Work out the finished part from the listing and answer in its coordinate system (mm). A direction names the side the tool comes from. Give positions to 0.01 mm unless a question says otherwise; leave off trailing zeros. Write each loop counter-clockwise with the first axis right and the second up, starting at its lowest first coordinate (ties: lowest second). Pieces come first, ordered by that corner, then holes. Notation, with made-up numbers: (65, 15.25) - (95, 15.25) arc R32 cw to (95, 50.25) - close; hole circle Ø1 at (89.5, -37). An arc over 180 degrees is marked (long way). Write item = value, one per line.
from build123d import *

# Parameters (mm, degrees)
PAD_DEPTH       = 25
SKETCH001_W     = 1
SKETCH001_H     = 8
SKETCH001_W_2   = 5
POCKET_DEPTH    = 14
SKETCH002_W     = 12.5
SKETCH002_H     = 8
POCKET001_DEPTH = 1.5
POCKET002_DEPTH = 0.5
SKETCH004_R     = 2
SKETCH004_W     = 0.8
SKETCH004_H     = 3
POCKET003_DEPTH = 8
SKETCH005_R     = 0.7
PAD001_DEPTH    = 2
SKETCH006_R     = 0.7
PAD002_DEPTH    = 2


with BuildPart() as part:
    # Sketch → Pad (new body, symmetric)
    with BuildSketch(Plane.YZ):
        with BuildLine():
            Line((-6, 13.5), (8, 13.5))
            Line((8, 13.5), (8, 0))
            Line((8, 0), (-8, 0))
            Line((-8, 0), (-8, 11.5))
            ThreePointArc((-6, 13.5), (-7.414214, 12.914214), (-8, 11.5))
        make_face()
    extrude(amount=PAD_DEPTH, both=True)

    # Sketch001 (on Face4 of Pad) → Pocket (cut)
    with BuildSketch(Plane(origin=(0, -8, 0), x_dir=(0, 0, -1), z_dir=(0, -1, 0))):
        with Locations((-0.5, -19)):
            Rectangle(SKETCH001_W, SKETCH001_H)
        with Locations((-0.5, -9.5)):
            Rectangle(SKETCH001_W, SKETCH001_H)
        with Locations((-0.5, 0)):
            Rectangle(SKETCH001_W, SKETCH001_H)
        with Locations((-0.5, 9.5)):
            Rectangle(SKETCH001_W, SKETCH001_H)
        with Locations((-0.5, 19)):
            Rectangle(SKETCH001_W, SKETCH001_H)
        with Locations((-11, -19)):
            Rectangle(SKETCH001_W_2, SKETCH001_H)
        with Locations((-11, -9.5)):
            Rectangle(SKETCH001_W_2, SKETCH001_H)
        with Locations((-11, 0)):
            Rectangle(SKETCH001_W_2, SKETCH001_H)
        with Locations((-11, 9.5)):
            Rectangle(SKETCH001_W_2, SKETCH001_H)
        with Locations((-11, 19)):
            Rectangle(SKETCH001_W_2, SKETCH001_H)
    extrude(amount=-POCKET_DEPTH, mode=Mode.SUBTRACT)

    # Sketch002 (on Face3 of Pocket) → Pocket001 (cut)
    with BuildSketch(Plane.ZX.offset(8)):
        with Locations((6.25, 19)):
            Rectangle(SKETCH002_W, SKETCH002_H)
        with Locations((6.25, 9.5)):
            Rectangle(SKETCH002_W, SKETCH002_H)
        with Locations((6.25, 0)):
            Rectangle(SKETCH002_W, SKETCH002_H)
        with Locations((6.25, -9.5)):
            Rectangle(SKETCH002_W, SKETCH002_H)
        with Locations((6.25, -19)):
            Rectangle(SKETCH002_W, SKETCH002_H)
    extrude(amount=-POCKET001_DEPTH, mode=Mode.SUBTRACT)

    # Sketch003 (on Face67 of Pocket001) → Pocket002 (cut)
    with BuildSketch(Plane.ZX.offset(6.5)):
        Polygon((0, 23), (8.5, 23), (8.5, 21.5), (9.5, 21.5), (9.5, 16.5), (8.5, 16.5), (8.5, 15), (0, 15), align=None)
        Polygon((0, 13.5), (8.5, 13.5), (8.5, 12), (9.5, 12), (9.5, 7), (8.5, 7), (8.5, 5.5), (0, 5.5), align=None)
        Polygon((0, 4), (8.5, 4), (8.5, 2.5), (9.5, 2.5), (9.5, -2.5), (8.5, -2.5), (8.5, -4), (0, -4), align=None)
        Polygon((0, -5.5), (8.5, -5.5), (8.5, -7), (9.5, -7), (9.5, -12), (8.5, -12), (8.5, -13.5), (0, -13.5), align=None)
        Polygon((0, -15), (8.5, -15), (8.5, -16.5), (9.5, -16.5), (9.5, -21.5), (8.5, -21.5), (8.5, -23), (0, -23), align=None)
    extrude(amount=-POCKET002_DEPTH, mode=Mode.SUBTRACT)

    # Sketch004 (on Face64 of Pocket002) → Pocket003 (cut)
    with BuildSketch(Plane(origin=(0, 0, 8.5), x_dir=(0, -1, 0), z_dir=(0, 0, 1))):
        with Locations((1.05, -19)):
            Circle(SKETCH004_R)
        with Locations((1.05, -9.5)):
            Circle(SKETCH004_R)
        with Locations((1.05, 0)):
            Circle(SKETCH004_R)
        with Locations((1.05, 9.5)):
            Circle(SKETCH004_R)
        with Locations((1.05, 19)):
            Circle(SKETCH004_R)
        with Locations((-4, -19)):
            Rectangle(SKETCH004_W, SKETCH004_H)
        with Locations((-4, -9.5)):
            Rectangle(SKETCH004_W, SKETCH004_H)
        with Locations((-4, 0)):
            Rectangle(SKETCH004_W, SKETCH004_H)
        with Locations((-4, 9.5)):
            Rectangle(SKETCH004_W, SKETCH004_H)
        with Locations((-4, 19)):
            Rectangle(SKETCH004_W, SKETCH004_H)
        with Locations((6.1, -19)):
            Rectangle(SKETCH004_W, SKETCH004_H)
        with Locations((6.1, -9.5)):
            Rectangle(SKETCH004_W, SKETCH004_H)
        with Locations((6.1, 0)):
            Rectangle(SKETCH004_W, SKETCH004_H)
        with Locations((6.1, 9.5)):
            Rectangle(SKETCH004_W, SKETCH004_H)
        with Locations((6.1, 19)):
            Rectangle(SKETCH004_W, SKETCH004_H)
    extrude(amount=-POCKET003_DEPTH, mode=Mode.SUBTRACT)

    # Sketch005 (on Face2 of Pocket003) → Pad001 (join)
    with BuildSketch(Plane(origin=(-25, 0, 0), x_dir=(0, 1, 0), z_dir=(-1, 0, 0))):
        with BuildLine():
            Line((-6, -13.5), (-2, -13.5))
            Line((-2, -13.5), (-2, -16.3))
            ThreePointArc((-2.7, -17), (-2.205025, -16.794975), (-2, -16.3))
            Line((-2.7, -17), (-5.3, -17))
            ThreePointArc((-6, -16.3), (-5.794975, -16.794975), (-5.3, -17))
            Line((-6, -16.3), (-6, -13.5))
        make_face()
        with Locations((-4, -15.5)):
            Circle(SKETCH005_R, mode=Mode.SUBTRACT)
        with BuildLine():
            Line((4, -13.5), (8, -13.5))
            Line((8, -13.5), (8, -16.3))
            ThreePointArc((7.3, -17), (7.794975, -16.794975), (8, -16.3))
            Line((7.3, -17), (4.7, -17))
            ThreePointArc((4, -16.3), (4.205025, -16.794975), (4.7, -17))
            Line((4, -16.3), (4, -13.5))
        make_face()
        with Locations((6, -15.5)):
            Circle(SKETCH005_R, mode=Mode.SUBTRACT)
    extrude(amount=-PAD001_DEPTH)

    # Sketch006 (on Face4 of Pocket003) → Pad002 (join)
    with BuildSketch(Plane(origin=(25, 0, 0), x_dir=(0, 1, 0), z_dir=(-1, 0, 0))):
        with BuildLine():
            Line((-6, -13.5), (-2, -13.5))
            Line((-2, -13.5), (-2, -16.3))
            ThreePointArc((-2.7, -17), (-2.205025, -16.794975), (-2, -16.3))
            Line((-2.7, -17), (-5.3, -17))
            ThreePointArc((-6, -16.3), (-5.794975, -16.794975), (-5.3, -17))
            Line((-6, -16.3), (-6, -13.5))
        make_face()
        with Locations((-4, -15.5)):
            Circle(SKETCH006_R, mode=Mode.SUBTRACT)
        with BuildLine():
            Line((4, -13.5), (8, -13.5))
            Line((8, -13.5), (8, -16.3))
            ThreePointArc((7.3, -17), (7.794975, -16.794975), (8, -16.3))
            Line((7.3, -17), (4.7, -17))
            ThreePointArc((4, -16.3), (4.205025, -16.794975), (4.7, -17))
            Line((4, -16.3), (4, -13.5))
        make_face()
        with Locations((6, -15.5)):
            Circle(SKETCH006_R, mode=Mode.SUBTRACT)
    extrude(amount=PAD002_DEPTH)


solid = part.part
1. Given pin 1 (2.5 mm diameter, centred on x = -19.5, y = -4, fed in from +Z); pin 2 (3 mm diameter, centred on x = 8.5, y = 4, fed in from -Z); pin 3 (6 mm diameter, centred on x = 0.5, z = 4.5, fed in from +Y), each flat-ended and moving along its own axis, determine where each tip first touches the part or whether it passes through.
Solution:
pin_1 = 8.5
pin_2 = 1
pin_3 = 6
2. Find section D-D, the plane z = 6.75. Give the number of separate pieces and of enclosed holes in the cut face, then the cut area to 3 significant figures.
Solution:
separate_pieces = 1
enclosed_holes = 15
area = 633 mm^2
3. A tool of negligible diameter and unlimited length cuts with its end or side. For faces 1 (the flat face through (15, 7, 3)), 2 (the flat face through (9, 4.4, 5)), 3 (the flat face through (15, -1, 11)), 4 (the flat face through (7.7, 0.5, 1)), from which of +Z, -Z, +X, -X, +Y, -Y can it reach the whole face along a straight path? Write none if from no direction.
Solution:
face_1 = -Z, +Y
face_2 = +Z, -Z
face_3 = +Z, -Y
face_4 = -Z, +Y, -Y
4. For a pull along Y with two mould halves and no side action, classify faces 5 (the flat face through (-19, 3.6, 5)), 6 (the cylindrical face through (24.01, -7.4, 12.93)), 7 (the flat face through (0, 7, 12.5)) as pulls with the +Y half, pulls with the -Y half, needs draft (parallel to the pull), parting line crosses it, or undercut.
Solution:
face_5 = undercut
face_6 = pulls with the -Y half
face_7 = needs draft
5. Straight lines are drawn through the part: line 1 (X direction, y = -0.75, z = 11); line 2 (Y direction, x = -23.4, z = 15.5); line 3 (X direction, y = -1.05, z = 3.25). For each, find the intervals that lie inside material, in ascending order.
Solution:
line_1 = -25 to -23, -15 to -13.5, -5.5 to -4, 4 to 5.5, 13.5 to 15, 23 to 25
line_2 = -6 to -4.7, -3.3 to -2, 4 to 5.3, 6.7 to 8
line_3 = -25 to -21, -17 to -11.5, -7.5 to -2, 2 to 7.5, 11.5 to 17, 21 to 25
6. Find section A-A, the plane x = 19. Give the vertices of the cut face in (y, z).
Solution:
outline = (-8, 1) - (-6.5, 1) - (-6.5, 8.5) - (-8, 8.5) - close; (-5.7, 1) - (-3.05, 1) - (-3.05, 8.5) - (-5.7, 8.5) - close; (0.95, 1) - (3.6, 1) - (3.6, 8.5) - (0.95, 8.5) - close; (4.4, 1) - (6, 1) - (6, 8.5) - (4.4, 8.5) - close; (6, 9.5) - (6.5, 9.5) - (6.5, 12.5) - (8, 12.5) - (8, 13.5) - (6, 13.5) - close
7. Find section B-B, the plane z = 14. Give the vertices of the cut face in (x, y), then the cut area to 3 significant figures.
Solution:
outline = (-25, -6) - (-23, -6) - (-23, -2) - (-25, -2) - close; (-25, 4) - (-23, 4) - (-23, 8) - (-25, 8) - close; (23, -6) - (25, -6) - (25, -2) - (23, -2) - close; (23, 4) - (25, 4) - (25, 8) - (23, 8) - close
area = 32.0 mm^2
